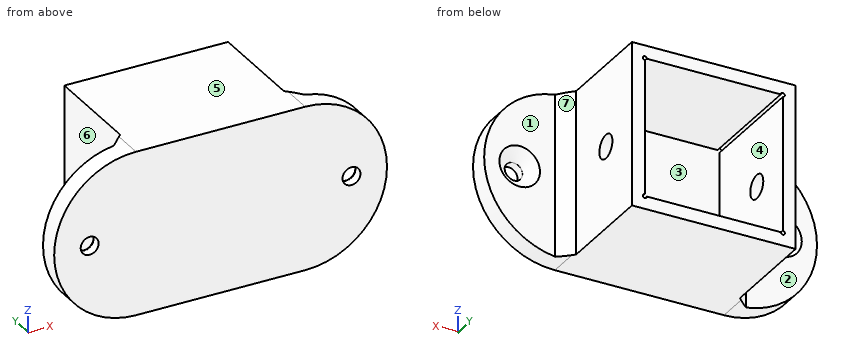
from build123d import *

# Parameters (mm, degrees)
BOSS_EXTRUDE1_DEPTH     = 3.81
SKETCH2_W               = 30.734
SKETCH2_H               = 30.734
SKETCH2_W_2             = 25.908
SKETCH2_H_2             = 25.908
BOSS_EXTRUDE2_DEPTH     = 21.59
CHAMFER1_SIZE           = 2.54
SKETCH3_R               = 1.68275
CUT_EXTRUDE1_DEPTH      = 3.81
CUT_EXTRUDE2_DEPTH      = 54.240878222
CUT_EXTRUDE2_DEPTH_BACK = 54.240878222
SKETCH6_R               = 2.2225
SKETCH8_R               = 0.381
CUT_EXTRUDE3_DEPTH      = 21.59


with BuildPart() as part:
    # Sketch1 → Boss-Extrude1 (new body)
    with BuildSketch(Plane(origin=(0, 0, 0), x_dir=(1, 0, 0), z_dir=(0, 1, 0))):
        with BuildLine():
            Line((-15.875, 15.367), (15.875, 15.367))
            ThreePointArc((15.875, 15.367), (31.242, 0), (15.875, -15.367))
            Line((15.875, -15.367), (-15.875, -15.367))
            ThreePointArc((-15.875, -15.367), (-31.242, 0), (-15.875, 15.367))
        make_face()
    extrude(amount=BOSS_EXTRUDE1_DEPTH)

    # Sketch2 → Boss-Extrude2 (add)
    with BuildSketch(Plane(origin=(0, 3.81, 0), x_dir=(1, 0, 0), z_dir=(0, 1, 0))):
        Rectangle(SKETCH2_W, SKETCH2_H)
        Rectangle(SKETCH2_W_2, SKETCH2_H_2, mode=Mode.SUBTRACT)
    extrude(amount=BOSS_EXTRUDE2_DEPTH)

    # Chamfer1
    chamfer1_edges = [part.edges().sort_by_distance(p)[0] for p in [
        (15.367, 3.81, 0),
        (-15.367, 3.81, 0),
    ]]
    chamfer(chamfer1_edges, length=CHAMFER1_SIZE)

    # Sketch3 → Cut-Extrude1 (cut)
    with BuildSketch(Plane(origin=(0, 3.81, 0), x_dir=(1, 0, 0), z_dir=(0, 1, 0))):
        with Locations(Location((-24.5745, 0, 0), (0, 0, 270))):
            Circle(SKETCH3_R)
        with Locations(Location((24.5745, 0, 0), (0, 0, 270))):
            Circle(SKETCH3_R)
    extrude(amount=-CUT_EXTRUDE1_DEPTH, mode=Mode.SUBTRACT)

    # Cut-Loft1: read off the stored shape, not the designer's step
    # Cut-Loft1: loft between two sections, ruled curve by curve
    cut_loft1_from = [
        Edge.make_bspline([(-26.145987116, 1.27, -0.601727352), (-27.349441821, 1.27, 2.54124688), (-24.206467589, 1.27, 3.744701584), (-23.003012884, 1.27, 0.601727352), (-21.799558179, 1.27, -2.54124688), (-24.942532411, 1.27, -3.744701584), (-26.145987116, 1.27, -0.601727352)], [0, 0, 0, 0, 0.5, 0.5, 0.5, 1, 1, 1, 1], 3, [1, 0.333333333, 0.333333333, 1, 0.333333333, 0.333333333, 1]),
    ]
    cut_loft1_to = [
        Edge.make_bspline([(-24.211181072, 3.81, -3.79263752), (-31.796456111, 3.81, -4.519275376), (-32.523093968, 3.81, 3.065999663), (-24.937818928, 3.81, 3.79263752), (-17.352543889, 3.81, 4.519275376), (-16.625906032, 3.81, -3.065999663), (-24.211181072, 3.81, -3.79263752)], [0, 0, 0, 0, 0.5, 0.5, 0.5, 1, 1, 1, 1], 3, [1, 0.333333333, 0.333333333, 1, 0.333333333, 0.333333333, 1]),
    ]
    cut_loft1 = Solid(Shell([*[Face.make_surface_from_curves(cut_loft1_from[k], cut_loft1_to[k]) for k in range(1)], Face(Wire(cut_loft1_from)), Face(Wire(cut_loft1_to))]))
    add(cut_loft1, mode=Mode.SUBTRACT)

    # Mirror1: Cut-Loft1 across plane
    add(cut_loft1.mirror(Plane(origin=(0, 0, 0), x_dir=(0, 0, 1), z_dir=(1, 0, 0))), mode=Mode.SUBTRACT)

    # Sketch6 → Cut-Extrude2 (cut, two sides: drawn at the far end of the back side and taken through both)
    with BuildSketch(Plane.ZY.offset(-12.954).offset(-CUT_EXTRUDE2_DEPTH_BACK)):
        with Locations(Location((0, 16.51, 0), (0, 0, 180))):
            Circle(SKETCH6_R)
    extrude(amount=CUT_EXTRUDE2_DEPTH + CUT_EXTRUDE2_DEPTH_BACK, mode=Mode.SUBTRACT)

    # Sketch8 → Cut-Extrude3 (cut)
    with BuildSketch(Plane(origin=(0, 25.4, 0), x_dir=(1, 0, 0), z_dir=(0, 1, 0))):
        with Locations((-12.954, 12.954)):
            Circle(SKETCH8_R)
        with Locations((12.954, 12.954)):
            Circle(SKETCH8_R)
        with Locations((12.954, -12.954)):
            Circle(SKETCH8_R)
        with Locations((-12.954, -12.954)):
            Circle(SKETCH8_R)
    extrude(amount=-CUT_EXTRUDE3_DEPTH, mode=Mode.SUBTRACT)


solid = part.part
Work out the finished part from the listing and answer in its coordinate system (mm). Face numbers are marked on the shaded views. A direction names the side the tool comes from. Give positions to 0.01 mm unless a question says otherwise; leave off trailing zeros. Write each loop counter-clockwise with the first axis right and the second up, starting at its lowest first coordinate (ties: lowest second). Pieces come first, ordered by that corner, then holes. Notation, with made-up numbers: (62.5, -22) - (96.5, -22) arc R17 ccw to (96.5, 7) - close; hole circle Ø6 at (31, -25). An arc over 180 degrees is marked (long way). One line per item, written item: value. Start each with the question number.
1. Given pin 1 (5.5 mm diameter, centred on x = -24.57, z = 0, fed in from +Y); pin 2 (2 mm diameter, centred on x = 24.57, z = 0, fed in from +Y); pin 3 (4 mm diameter, centred on x = -21.5, z = 0.5, fed in from +Y); pin 4 (10 mm diameter, centred on y = 9, z = 5.5, fed in from -X), each flat-ended and moving along its own axis, determine where each tip first touches the part or whether it passes through.
2. Consider probe 1 along X at (y, z) = (0.5, 0); probe 2 along X at (y, z) = (22.75, 13); probe 3 along X at (y, z) = (13, 10). Determine where each line is inside the solid, lowest interval first.
3. Find section A-A (y = 16.51). Write down the section's boundary in (x, z), then the cut area to 3 significant figures.
4. Find section C-C (x = 5.5). Write down the section's boundary in (y, z), then the cut area to 3 significant figures.
5. For the marked faces 1, 2 and 3, determine the directions among +Z, -Z, +X, -X, +Y, -Y from which every point of the face is accessible in a straight line to the end or side of a thin tool.
6. Find section B-B (y = 12.5). Write down the section's boundary in (x, z).
7. Find section D-D (z = 0). State how many separate pieces and enclosed holes the cut face has, then the cut area to 3 significant figures.
8. For a pull along X with two mould halves and no side action, classify the marked faces 4, 5, 6 and 7 as +X half, -X half, draft (parallel to the pull), parting line (faces both ways), or undercut.
Geometry results:
1. pin 1: y = 2.97
1. pin 2: through
1. pin 3: y = 3.81
1. pin 4: x = -17.72
2. probe 1: -31.24 to -26.26, -22.89 to 22.89, 26.26 to 31.24
2. probe 2: -15.37 to -13.33, -12.58 to 12.58, 13.33 to 15.37
2. probe 3: -15.37 to -12.95, 12.95 to 15.37
3. outline: (-15.37, -15.37) - (15.37, -15.37) - (15.37, -2.22) - (12.95, -2.22) - (12.95, -12.57) arc R0.38 cw (long way) to (12.57, -12.95) - (-12.57, -12.95) arc R0.38 cw (long way) to (-12.95, -12.57) - (-12.95, -2.22) - (-15.37, -2.22) - close; (-15.37, 2.22) - (-12.95, 2.22) - (-12.95, 12.57) arc R0.38 cw (long way) to (-12.57, 12.95) - (12.57, 12.95) arc R0.38 cw (long way) to (12.95, 12.57) - (12.95, 2.22) - (15.37, 2.22) - (15.37, 15.37) - (-15.37, 15.37) - close
3. area: 251 mm2
4. outline: (0, -15.37) - (25.4, -15.37) - (25.4, -12.95) - (3.81, -12.95) - (3.81, 12.95) - (25.4, 12.95) - (25.4, 15.37) - (0, 15.37) - close
4. area: 221 mm2
5. face 1: +Z, -Z, +X, +Y
5. face 2: +Z, -Z, -X, +Y
5. face 3: +Y
6. outline: (-15.37, -15.37) - (15.37, -15.37) - (15.37, 15.37) - (-15.37, 15.37) - close; hole (-12.95, -12.57) arc R0.38 ccw (long way) to (-12.57, -12.95) - (12.57, -12.95) arc R0.38 ccw (long way) to (12.95, -12.57) - (12.95, 12.57) arc R0.38 ccw (long way) to (12.57, 12.95) - (-12.57, 12.95) arc R0.38 ccw (long way) to (-12.95, 12.57) - close
7. separate pieces: 5
7. enclosed holes: 0
7. area: 294 mm2
8. face 4: undercut
8. face 5: draft
8. face 6: -X half
8. face 7: +X half
